Read the model definition and answer for the solid it produces. Units are mm, in the model's axes. A direction names the side the tool comes from. Give positions to 0.01 mm unless a question says otherwise; leave off trailing zeros. Order: outer loops, then holes, each group sorted by start corner. A loop starts at its lowest first (then second) coordinate and runs counter-clockwise, first axis right, second up.
Item 1: A cutting plane is placed at A-A (y = -3.5). State how many separate pieces and enclosed holes the cut face has, plus the area to 3 significant figures.
Item 2: Find the intervals of material crossed by line 1 along Z through (x, y) = (0, -2.65) (3 decimals); line 2 along X through (y, z) = (-1, 2); line 3 along X through (y, z) = (-2.5, 1), in increasing order.
Item 3: Which of the six approach directions +Z, -Z, +X, -X, +Y, -Y give full straight-line access (tool end or side, diameter ignored) to faces 1 (the face through (-2, 11.43, 0)), 2 (the face through (0, 0, 0))?
Item 4: The mould has two halves that part along X. Classify faces 3 (the face through (-2.54, -2.19, -5.38)), 4 (the face through (0, -4.318, 0)), 5 (the face through (0.83, 5.63, -3.72)): +X half, -X half, draft (parallel to the pull), parting line (faces both ways), or undercut.
Item 5: A cutting plane is placed at C-C (y = 3.25). Write down the section's boundary in (x, z) (1 decimal), plus the area to 3 significant figures.
Item 6: Given pin 1 Ø2.5 at (x, z) = (0, 0) entering from +Y; pin 2 Ø3.5 at (x, z) = (0, 7.62) entering from +Y, each flat-ended and moving along its own axis, determine where each tip first touches the part or whether it passes through.
from build123d import *

# Parameters (mm, degrees)
F0_R     = 16.764
F1_DEPTH = 4.318
F2_R     = 1.5875
F3_R     = 1.905
F4_DEPTH = 25.4
F5_R     = 1.5875
F6_DEPTH = 19.05
F5_R_2   = 3.81
F7_DEPTH = 11.43


with BuildPart() as f1:
    # F0 (on Front) → F1 (new body)
    with BuildSketch(Plane.XZ):
        Circle(F0_R)
    extrude(amount=F1_DEPTH)

    # F2
    f2_edges = [f1.edges().sort_by_distance(p)[0] for p in [
        (-16.764, 0, 0),
        (-16.764, -4.318, 0),
    ]]
    fillet(f2_edges, radius=F2_R)

    # F3 (on face) → F4 (cut)
    with BuildSketch(Plane.XZ.offset(4.318)):
        with BuildLine():
            ThreePointArc((0, 5.715), (1.347038, 6.272962), (1.905, 7.62))
            ThreePointArc((1.905, 7.62), (-1.347038, 8.967038), (0, 5.715))
        make_face()
        with Locations((4.370652, 6.241939)):
            Circle(F3_R)
        with Locations((7.439376, 1.64927)):
            Circle(F3_R)
        with Locations((6.599114, -3.81)):
            Circle(F3_R)
        with Locations((3.220351, -6.906065)):
            Circle(F3_R)
        with Locations((-2.291378, -7.267323)):
            Circle(F3_R)
        with Locations((-6.599114, -3.81)):
            Circle(F3_R)
        with Locations((-7.591004, 0.664127)):
            Circle(F3_R)
        with Locations((-5.147997, 5.618053)):
            Circle(F3_R)
    extrude(amount=-F4_DEPTH, mode=Mode.SUBTRACT)

    # F5 (on face) → F6 (cut)
    with BuildSketch(Plane(origin=(0, 0, 0), x_dir=(-1, 0, 0), z_dir=(0, 1, 0))):
        Circle(F5_R)
    extrude(amount=F6_DEPTH, mode=Mode.SUBTRACT)

    # F5 (on face) → F7 (join)
    with BuildSketch(Plane(origin=(0, 0, 0), x_dir=(-1, 0, 0), z_dir=(0, 1, 0))):
        Circle(F5_R_2)
        Circle(F5_R, mode=Mode.SUBTRACT)
    extrude(amount=F7_DEPTH)


solid = f1.part
Response values:
1. separate pieces: 1
1. enclosed holes: 9
1. area: 759 mm2
2. line 1: z = -16.764 to 5.715, 9.525 to 16.764
2. line 2: x = -16.53 to -8.95, -6.23 to 5.57, 9.31 to 16.53
2. line 3: x = -16.73 to -9.47, -5.72 to 5.65, 9.23 to 16.73
3. face 1: +Z, -Z, +X, -X, +Y
3. face 2: +Y
4. face 3: undercut
4. face 4: draft
4. face 5: parting line
5. outline: circle Ø7.6 at (0, 0); hole circle Ø3.2 at (0, 0)
5. area: 37.7 mm2
6. pin 1: stops at y = 0
6. pin 2: passes through
